from build123d import *

# Parameters (mm, degrees)
FILLET1_R               = 10
FILLET2_R               = 10
CUT_EXTRUDE1_DEPTH      = 113.630542396
CUT_EXTRUDE1_DEPTH_BACK = 113.630542396
SKETCH2_W               = 43
SKETCH2_H               = 10


with BuildPart() as part:
    # Sketch1 → Revolve1 (revolve)
    with BuildSketch(Plane(origin=(0, 0, 0), x_dir=(1, 0, 0), z_dir=(0, 1, 0))):
        Polygon((-99.363670728, 9.691024676), (-63.789023183, 9.691024676), (-63.789023183, 25), (24.210976817, 25), (24.210976817, 37.5), (36.210976817, 37.5), (36.210976817, 20), (-29.789023183, 20), (-29.789023183, 0), (-99.363670728, 0), align=None)
    revolve(axis=Axis((-29.789023183, 0, 0), (-1, 0, 0)))

    # Fillet1
    fillet1_edges = [part.edges().sort_by_distance(p)[0] for p in [
        (-63.789023183, 0, 25),
    ]]
    fillet(fillet1_edges, radius=FILLET1_R)

    # Fillet2
    fillet2_edges = [part.edges().sort_by_distance(p)[0] for p in [
        (-63.789023183, 0, 9.691024676),
    ]]
    fillet(fillet2_edges, radius=FILLET2_R)

    # Sketch2 → Cut-Extrude1 (cut, two sides: drawn at the far end of the back side and taken through both)
    with BuildSketch(Plane(origin=(0, 0, 0), x_dir=(1, 0, 0), z_dir=(0, 1, 0)).offset(-CUT_EXTRUDE1_DEPTH_BACK)):
        with Locations((2.710976817, -0.126659564)):
            Rectangle(SKETCH2_W, SKETCH2_H)
    extrude(amount=CUT_EXTRUDE1_DEPTH + CUT_EXTRUDE1_DEPTH_BACK, mode=Mode.SUBTRACT)


solid = part.part
The model under review builds one solid part; all positions refer to its coordinate system, in mm. A direction names the side the tool comes from. Coordinates: 2 decimals unless noted, no trailing zeros. Order: outer loops, then holes, each group sorted by start corner. A loop starts at its lowest first (then second) coordinate and runs counter-clockwise, first axis right, second up. Notation, with made-up numbers: (60, -14.75) -> (71, -14.75) arc R35 ccw to (71, 19.25) -> close; hole circle Ø9 at (-27, 61.25). An arc over 180 degrees is marked (long way). Answer in a Markdown table with one row per item.
(1) Consider section D-D (y = -27). Write out the cut boundary in (x, z).
Answers:
| item | result |
|---|---|
| outline | (24.21, -26.02) -> (36.21, -26.02) -> (36.21, 26.02) -> (24.21, 26.02) -> close |
(2) Consider section B-B (z = -1). State how many separate pieces and enclosed holes the cut face has, plus the area to 3 significant figures.
Answers:
| item | result |
|---|---|
| separate pieces | 3 |
| enclosed holes | 0 |
| area | 2,910 mm² |
(3) The part is to be moulded in two halves that separate along Z. For faces 1 (the flat face through (-99.364, 0, 0)), 2 (the cylindrical face through (30.29, -37.18, 4.88)), 3 (the flat face through (-18.789, 22, 0)), say which applies: +Z half, -Z half, draft (parallel to the pull), parting line (faces both ways), or undercut.
Answers:
| item | result |
|---|---|
| face 1 | draft |
| face 2 | parting line |
| face 3 | undercut |
(4) Consider section A-A (x = 5.5). Write out the cut boundary in (y, z).
Answers:
| item | result |
|---|---|
| outline | (-24.52, -4.87) arc R25 ccw to (24.52, -4.87) -> (19.4, -4.87) arc R20 cw to (-19.4, -4.87) -> close; (-24.47, 5.13) -> (-19.33, 5.13) arc R20 cw to (19.33, 5.13) -> (24.47, 5.13) arc R25 ccw to start |
(5) Wall thickness on line 1 along Z through (x, y) = (14, 0); line 2 along X through (y, z) = (-30.5, -19); line 3 along Y through (x, z) = (-25.5, 11): over which ranges is each line inside the solid? List them lowest first.
Answers:
| item | result |
|---|---|
| line 1 | -25 to -20, 20 to 25 |
| line 2 | 24.21 to 36.21 |
| line 3 | -22.45 to -16.7, 16.7 to 22.45 |
(6) Machinability: for faces 4 (the flat face through (-29.789, 0, 0)), 5 (the flat face through (2, 22, 5.127)), 6 (the cylindrical face through (-14.2, 22.2, -11.5)), 7 (the flat face through (36.211, 16, -16)), which of the approach directions +Z, -Z, +X, -X, +Y, -Y give a long, thin tool a straight path to every point of the face, cutting with its end or side? Answer none if there is none.
Answers:
| item | result |
|---|---|
| face 4 | +X |
| face 5 | +Y, -Y |
| face 6 | -X |
| face 7 | +Z, -Z, +X, +Y, -Y |
(7) Consider section C-C (x = -39). Write out the cut boundary in (y, z), plus the area to 3 significant figures.
Answers:
| item | result |
|---|---|
| outline | circle Ø50 at (0, 0) |
| area | 1,960 mm² |
(8) Insertion check: pin 1 (12 mm diameter, centred on x = 12, y = 2.5, fed in from +Z); pin 2 (2 mm diameter, centred on x = -16, z = 10.5, fed in from -Y); pin 3 (12 mm diameter, centred on x = -58.5, z = 3, fed in from +Y). Each pin has a flat end and moves straight along its axis. Give the tip position at first contact, or say it passes through.
Answers:
| item | result |
|---|---|
| pin 1 | z = 25 |
| pin 2 | y = -23.12 |
| pin 3 | y = 25 |
